CAD build for the part. Positions are in the model's coordinates, mm. A direction names the side the tool comes from. Give positions to 0.01 mm unless a question says otherwise; leave off trailing zeros. Order: outer loops, then holes, each group sorted by start corner. A loop starts at its lowest first (then second) coordinate and runs counter-clockwise, first axis right, second up. Notation, with made-up numbers: (14.5, -27.5) -> (71.5, -27.5) arc R12 cw to (71.5, -22.5) -> close; hole circle Ø7 at (31, 48.5). An arc over 180 degrees is marked (long way). Answer as CSV lines item,"result".
```python
from build123d import *

# Parameters (mm, degrees)
SKETCH_1_W          = 14
SKETCH_1_H          = 7
SKETCH_2_W          = 62
SKETCH_2_H          = 3
SKETCH_3_R          = 4
CUT_EXTRUDE_1_DEPTH = 35.727510858
SKETCH_5_R          = 5
CUT_EXTRUDE_2_DEPTH = 3


with BuildPart() as part:
    # 草图1 → 旋转1 (revolve)
    with BuildSketch(Plane.XY, mode=Mode.PRIVATE) as revolve_1_sk:
        with Locations((0, 3.5)):
            Rectangle(SKETCH_1_W, SKETCH_1_H)
    revolve(revolve_1_sk.sketch.rotate(Axis((-7, 0, 0), (1, 0, 0)), 90), axis=Axis((-7, 0, 0), (1, 0, 0)))

    # 草图2 → 旋转3 (revolve)
    with BuildSketch(Plane(origin=(0, 0, 0), x_dir=(0, 0, -1), z_dir=(1, 0, 0)), mode=Mode.PRIVATE) as revolve_3_sk:
        with Locations((0, 1.5)):
            Rectangle(SKETCH_2_W, SKETCH_2_H)
    revolve(revolve_3_sk.sketch.rotate(Axis((0, 0, 31), (0, 0, -1)), 90), axis=Axis((0, 0, 31), (0, 0, -1)))

    # 草图3 → 切除-拉伸1 (cut, through all)
    with BuildSketch(Plane(origin=(7, 0, 0), x_dir=(0, 0, -1), z_dir=(1, 0, 0))):
        Circle(SKETCH_3_R)
    extrude(amount=-CUT_EXTRUDE_1_DEPTH, mode=Mode.SUBTRACT)

    # 草图5 → 切除-拉伸2 (cut)
    with BuildSketch(Plane(origin=(7, 0, 0), x_dir=(0, 0, -1), z_dir=(1, 0, 0))):
        Circle(SKETCH_5_R)
    cut_extrude_2 = extrude(amount=-CUT_EXTRUDE_2_DEPTH, mode=Mode.SUBTRACT)

    # 镜向1: 切除-拉伸2 across plane
    add(cut_extrude_2.mirror(Plane(origin=(0, 0, 0), x_dir=(0, 0, 1), z_dir=(1, 0, 0))), mode=Mode.SUBTRACT)


solid = part.part
```
1) Band-saw the part on A-A, the plane y = 0. Write the cut outline in (x, z), then the cut area to 3 significant figures.
Data:
outline,"(-7, -7) -> (-3, -7) -> (-3, -31) -> (3, -31) -> (3, -7) -> (7, -7) -> (7, -5) -> (4, -5) -> (4, -4) -> (-4, -4) -> (-4, -5) -> (-7, -5) -> close; (-7, 5) -> (-4, 5) -> (-4, 4) -> (4, 4) -> (4, 5) -> (7, 5) -> (7, 7) -> (3, 7) -> (3, 31) -> (-3, 31) -> (-3, 7) -> (-7, 7) -> close"
area,"360 mm2"
2) Band-saw the part on C-C, the plane z = 0. Write the cut outline in (x, y), then the cut area to 3 significant figures.
Data:
outline,"(-7, -7) -> (7, -7) -> (7, -5) -> (4, -5) -> (4, -4) -> (-4, -4) -> (-4, -5) -> (-7, -5) -> close; (-7, 5) -> (-4, 5) -> (-4, 4) -> (4, 4) -> (4, 5) -> (7, 5) -> (7, 7) -> (-7, 7) -> close"
area,"72.0 mm2"
3) Wall check: line 1 along Z through (x, y) = (0.5, -0.25); line 2 along Y through (x, z) = (5.85, 0); line 3 along X through (y, z) = (-3.25, 3). Give the ranges that are in metal, low to high. Write a range as [from, to].
Data:
line 1,"z = [-31, -3.99], [3.99, 31]"
line 2,"y = [-7, -5], [5, 7]"
line 3,"x = [-4, 4]"
4) Band-saw the part on B-B, the plane x = 0. Write the cut outline in (y, z).
Data:
outline,"(-3, -31) -> (3, -31) -> (3, -6.32) arc R7 ccw to (3, 6.32) -> (3, 31) -> (-3, 31) -> (-3, 6.32) arc R7 ccw to (-3, -6.32) -> close; hole circle Ø8 at (0, 0)"
5) Band-saw the part on D-D, the plane z = -19. Write the cut outline in (x, y), then the cut area to 3 significant figures.
Data:
outline,"circle Ø6 at (0, 0)"
area,"28.3 mm2"
6) Which spindle directions (+Z, -Z, +X, -X, +Y, -Y) get a long thin tool onto all of the face, cutting with end or side? Do faces 1 (the cylindrical face through (5.52, -4.88, 1.08)), 2 (the cylindrical face through (0.098, 4.259, -5.555)), 3 (the cylindrical face through (2.86, -0.9, -18.84)), 4 (the flat face through (7, -5, 2)). Say none if no direction does.
Data:
face 1,"+X"
face 2,"none"
face 3,"-Z"
face 4,"+Z, -Z, +X, +Y, -Y"
7) Pull direction Y, two halves, no side cores. Call faces 5 (the cylindrical face through (-5.52, -4.88, 1.08)), 6 (the cylindrical face through (2.86, -0.9, 18.49)), 7 (the flat face through (0, 0, 31)): pulls with the +Y half, pulls with the -Y half, needs draft (parallel to the pull), parting line crosses it, or undercut.
Data:
face 5,"undercut"
face 6,"parting line crosses it"
face 7,"needs draft"
8) Pin check, flat tips, straight feed: P1, Ø6, axis at x = -2.5, z = -9.5, coming from the +Y side; P2, Ø1, axis at x = 3, z = 12, coming from the +Y side; P3, Ø2, axis at y = 2, z = -23, coming from the +X side. Stop position of each tip, or through.
Data:
P1,"stops at y = 3"
P2,"stops at y = 1.66"
P3,"stops at x = 2.83"
